Could you check a few things on this model? Use its own coordinates, in mm. A direction names the side the tool comes from. Give positions to 0.01 mm unless a question says otherwise; leave off trailing zeros. Order: outer loops, then holes, each group sorted by start corner. A loop starts at its lowest first (then second) coordinate and runs counter-clockwise, first axis right, second up. Notation, with made-up numbers: M -9.75,36.5 L 20.25,36.5 A19 cw 20.25,67.5 Z; hole C 56,69 d6. An arc over 180 degrees is marked long. Answer in a Markdown table with one row per item. Add a question column.
Autodesk Inventor part; units mm, degrees
ref_plane "YZ Plane" through (0, 0, 0) normal (1, 0, 0) x (0, 1, 0)
ref_plane "XZ Plane" through (0, 0, 0) normal (0, 1, 0) x (-1, 0, 0)
ref_plane "XY Plane" through (0, 0, 0) normal (0, 0, 1) x (1, 0, 0)
sketch "Sketch1" plane through (0, 0, 0) normal (0, 1, 0) x (-1, 0, 0)
  line L0 (-1.27, 1.27) -> (1.27, 1.27)
  line L1 (1.27, 1.27) -> (1.27, -1.27)
  line L2 (1.27, -1.27) -> (-1.27, -1.27)
  line L3 (-1.27, -1.27) -> (-1.27, 1.27)
  line L4 (-1.27, 1.27) -> (1.27, -1.27) construction
  line L5 (1.27, 1.27) -> (-1.27, -1.27) construction
  line L6 (1.27, -1.27) -> (3.81, -1.27)
  line L7 (3.81, -1.27) -> (3.81, 1.27)
  line L8 (3.81, 1.27) -> (1.27, 1.27)
  line L9 (1.27, 1.27) -> (1.27, -1.27)
  point P0 (0, 0)
  dimension "d0" = 2.54
  dimension "d1" = 2.54
extrude "Extrusion1" add sketch "Sketch1" along normal blind 8.5
sketch "Sketch2" plane through (0, 8.5, 0) normal (0, 1, 0) x (1, 0, 0)
  line L0 (0.2, -0.2) -> (-0.2, -0.2)
  line L1 (-0.2, -0.2) -> (-0.2, 0.2)
  line L2 (-0.2, 0.2) -> (0.2, 0.2)
  line L3 (0.2, 0.2) -> (0.2, -0.2)
  line L4 (0.2, -0.2) -> (-0.2, 0.2) construction
  line L5 (-0.2, -0.2) -> (0.2, 0.2) construction
  line L6 (-2.34, 0.2) -> (-2.74, 0.2)
  line L7 (-2.74, 0.2) -> (-2.74, -0.2)
  line L8 (-2.74, -0.2) -> (-2.34, -0.2)
  line L9 (-2.34, -0.2) -> (-2.34, 0.2)
  line L10 (-2.34, 0.2) -> (-2.74, -0.2) construction
  line L11 (-2.74, 0.2) -> (-2.34, -0.2) construction
  point P0 (0, 0)
  point P1 (-2.54, 0)
  dimension "d4" = 0.4
  dimension "d5" = 0.4
  dimension "d45" = 0.4
  dimension "d46" = 2.54
extrude "Extrusion2" cut sketch "Sketch2" against normal blind 5
chamfer "Chamfer1" distance 0.75 angle 45 8 edges at (0, 8.5, 0.2) (-0.2, 8.5, 0) (0, 8.5, -0.2) (0.2, 8.5, 0) (-2.54, 8.5, -0.2) (-2.74, 8.5, 0) (-2.54, 8.5, 0.2) (-2.34, 8.5, 0)
sketch "Sketch3" plane through (0, 0, 0) normal (0, -1, 0) x (1, 0, 0)
  line L0 (-0.2, 0.2) -> (0.2, 0.2)
  line L1 (0.2, 0.2) -> (0.2, -0.2)
  line L2 (0.2, -0.2) -> (-0.2, -0.2)
  line L3 (-0.2, -0.2) -> (-0.2, 0.2)
  line L4 (-0.2, 0.2) -> (0.2, -0.2) construction
  line L5 (0.2, 0.2) -> (-0.2, -0.2) construction
  point P0 (0, 0)
  dimension "d11" = 0.4
  dimension "d12" = 0.4
extrude "Extrusion3" add sketch "Sketch3" along normal blind 1.5
sketch "Sketch4" plane through (-0.2, 0, 0.2) normal (0, 0, 1) x (1, 0, 0)
  line L0 (0, -1.5) -> (4.75, -1.5)
  line L1 (4.75, -1.5) -> (4.75, -1.1)
  line L2 (4.75, -1.1) -> (0, -1.1)
  line L3 (0, -1.1) -> (0, -1.5)
  point P0 (0.2, 0)
  dimension "d27" = 0.4
  dimension "d28" = 4.75
extrude "Extrusion4" add sketch "Sketch4" against normal up to surface (0.4 mm away)
fillet "Fillet1" radius 0.5 1 edges at (-0.2, -1.5, 0)
fillet "Fillet2" radius 0.15 1 edges at (0.2, -1.1, 0)
chamfer "Chamfer6" distance 0.5 distance2 0.1 1 edges at (4.55, -1.3, 0.2) measured on face at (1.7333, -1.3667, 0.2)
chamfer "Chamfer7" distance 0.5 distance2 0.1 1 edges at (4.55, -1.1, -0.05) measured on face at (2.9833, -1.1, -0.0667)
chamfer "Chamfer8" distance 0.1 distance2 0.5 1 edges at (4.55, -1.35, -0.2) measured on face at (4.55, -1.4, 0)
chamfer "Chamfer9" distance 0.1 distance2 0.5 1 edges at (4.55, -1.5, 0) measured on face at (4.55, -1.4, 0.0333)
sketch "Sketch5" plane through (0, 0, 0) normal (0, -1, 0) x (1, 0, 0)
  line L0 (-2.74, -0.2) -> (-2.34, -0.2)
  line L1 (-1.59, 0.95) -> (-2.34, 0.2)
  line L2 (-2.74, -0.2) -> (-2.34, -0.2)
  line L3 (-2.34, -0.2) -> (-2.34, 0.2)
  line L4 (-2.34, 0.2) -> (-2.74, 0.2)
  line L5 (-2.74, 0.2) -> (-2.74, -0.2)
  point P0 (0, 0)
extrude "Extrusion5" add sketch "Sketch5" along normal blind 4.04
sketch "Sketch6" plane through (-2.34, 0, -0.2) normal (0, 0, -1) x (-1, 0, 0)
  line L0 (0.4, 0) -> (0.4, -4.04)
  line L1 (0.4, -4.04) -> (-6.89, -4.04)
  line L2 (-6.89, -4.04) -> (-6.89, -3.64)
  line L3 (-6.89, -3.64) -> (0.4, -3.64)
  line L4 (0.4, -3.64) -> (0.4, -4.04)
  point P0 (-2.34, 0)
  dimension "d49" = 0.4
extrude "Extrusion6" add sketch "Sketch6" against normal up to surface (0.4 mm away)
fillet "Fillet3" radius 0.5 1 edges at (-2.74, -4.04, 0)
fillet "Fillet4" radius 0.15 1 edges at (-2.34, -3.64, 0)
chamfer "Chamfer10" distance 0.1 distance2 0.5 1 edges at (4.55, -3.84, 0.2) measured on face at (4.55, -3.7733, -0.0667)
chamfer "Chamfer11" distance 0.1 distance2 0.5 1 edges at (4.55, -3.64, -0.05) measured on face at (4.55, -3.7733, -0.1)
chamfer "Chamfer12" distance 0.5 distance2 0.1 1 edges at (4.55, -4.04, -0.05) measured on face at (2.12, -4.04, -0.0667)
chamfer "Chamfer13" distance 0.5 distance2 0.1 1 edges at (4.55, -3.84, -0.2) measured on face at (-0.1267, -3.9067, -0.2)
properties part number "FemaleHederPin_2_90"
1. Will these pins go through, and if not, where does the flat tip stop? P1, Ø1.6, axis at x = 1, y = -1, coming from the +Z side; P2, Ø1.6, axis at x = 2, y = -1, coming from the -Z side; P3, Ø4, axis at x = 2.5, y = 2, coming from the +Z side.
2. Suppose I cut it at B-B on x = 2.75. List the corners of the cut face in (y, z) for me, plus the area to 3 significant figures.
3. Suppose I cut it at A-A on y = -0.25. List the corners of the cut face in (x, z) for me, plus the area to 3 significant figures.
4. If I drill on line 1 along X through (y, z) = (5, 0); line 2 along X through (y, z) = (5, -0.35); line 3 along Y through (x, z) = (0.5, 0.1), over which ranges is the centre line in solid material (lowest first)? Write a range as [from, to].
5. For faces 1 (the flat face through (1.6, -1.3, -0.2)), 2 (the flat face through (-1, 4, 1.27)), 3 (the flat face through (-0.3, -3.8, 0.2)), which set-ups out of +Z, -Z, +X, -X, +Y, -Y let a thin tool reach every point of the face, with its end or its side?
6. Suppose I cut it at C-C on y = 5.25. List the corners of the cut face in (x, z) for me.
7. Suppose I cut it at D-D on z = -0.8. List the corners of the cut face in (x, y) for me.
Findings below:
| question | item | result |
|---|---|---|
| 1 | P1 | z = 0.2 |
| 1 | P2 | z = -0.2 |
| 1 | P3 | z = 1.27 |
| 2 | outline | M -4.04,-0.2 L -3.64,-0.2 L -3.64,0.2 L -4.04,0.2 Z; M -1.5,-0.2 L -1.1,-0.2 L -1.1,0.2 L -1.5,0.2 Z |
| 2 | area | 0.320 mm2 |
| 3 | outline | M -2.74,-0.2 L -2.34,-0.2 L -2.34,0.2 L -2.74,0.2 Z; M -0.2,-0.2 L 0.2,-0.2 L 0.2,0.2 L -0.2,0.2 Z |
| 3 | area | 0.320 mm2 |
| 4 | line 1 | [-3.81, -2.74], [-2.34, -0.2], [0.2, 1.27] |
| 4 | line 2 | [-3.81, 1.27] |
| 4 | line 3 | [-4.04, -3.64], [-1.5, -1.1], [0, 8.05] |
| 5 | face 1 | -Z, +X, -X, -Y |
| 5 | face 2 | +Z, +X, -X, +Y, -Y |
| 5 | face 3 | +Z, +X, -X, -Y |
| 6 | outline | M -3.81,-1.27 L 1.27,-1.27 L 1.27,1.27 L -3.81,1.27 Z; hole M -2.74,-0.2 L -2.34,-0.2 L -2.34,0.2 L -2.74,0.2 Z; hole M -0.2,-0.2 L 0.2,-0.2 L 0.2,0.2 L -0.2,0.2 Z |
| 7 | outline | M -3.81,0 L 1.27,0 L 1.27,8.5 L 0.95,8.5 L 0.8,8.35 L -0.8,8.35 L -0.95,8.5 L -1.59,8.5 L -1.74,8.35 L -3.34,8.35 L -3.49,8.5 L -3.81,8.5 Z |
